Geometry check sheet. Reference: drawing and pictorial views, mm from the part's lowest x, y, z. A direction names the side the tool comes from. Round coordinates to 2 decimals unless told otherwise and drop trailing zeros. Write each loop counter-clockwise with the first axis right and the second up, starting at its lowest first coordinate (ties: lowest second). Pieces come first, ordered by that corner, then holes. Notation, with made-up numbers: (14.25, 5.25) -> (55.25, 5.25) arc R14 ccw to (55.25, 12.25) -> close; hole circle Ø8 at (-1.75, 4.5). An arc over 180 degrees is marked (long way). Write item = value, one per line.
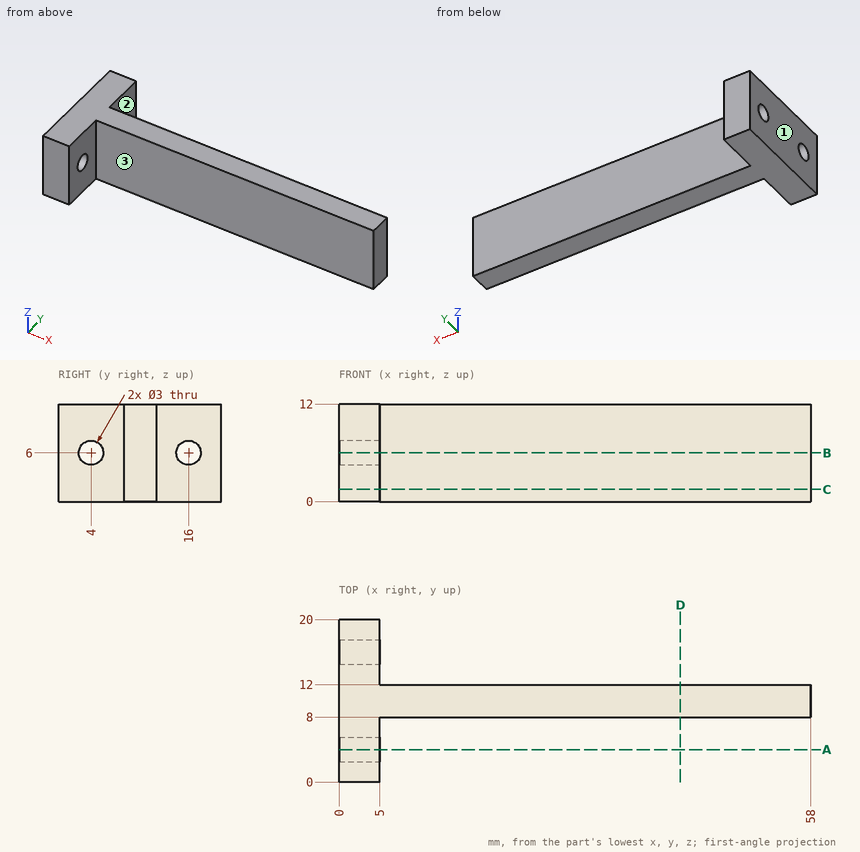
(1) Go/stop test with flat-tipped pins: P1, Ø1.5, axis at x = 44.5, z = 7.5, coming from the -Y side; P2, Ø6.5, axis at y = 2.5, z = 4, coming from the +X side; P3, Ø1, axis at y = 16.5, z = 6, coming from the +X side; P4, Ø6, axis at x = 21.5, z = 5.5, coming from the +Y side. Record where each tip stops, or that it passes through.
Worked answers:
P1 = 8
P2 = 5
P3 = through
P4 = 12
(2) Sectioned sample at D-D on x = 42. Enter the section's corners in (y, z), then the cut area to 3 significant figures.
Worked answers:
outline = (8, 0) -> (12, 0) -> (12, 12) -> (8, 12) -> close
area = 48.0 mm²
(3) Sectioned sample at A-A on y = 4. Enter the section's corners in (x, z).
Worked answers:
outline = (0, 0) -> (5, 0) -> (5, 4.5) -> (0, 4.5) -> close; (0, 7.5) -> (5, 7.5) -> (5, 12) -> (0, 12) -> close
(4) Sectioned sample at C-C on z = 1.5. Enter the section's corners in (x, y), then the cut area to 3 significant figures.
Worked answers:
outline = (0, 0) -> (5, 0) -> (5, 8) -> (58, 8) -> (58, 12) -> (5, 12) -> (5, 20) -> (0, 20) -> close
area = 312 mm²
(5) Sectioned sample at B-B on z = 6. Enter the section's corners in (x, y).
Worked answers:
outline = (0, 0) -> (5, 0) -> (5, 2.5) -> (0, 2.5) -> close; (0, 5.5) -> (5, 5.5) -> (5, 8) -> (58, 8) -> (58, 12) -> (5, 12) -> (5, 14.5) -> (0, 14.5) -> close; (0, 17.5) -> (5, 17.5) -> (5, 20) -> (0, 20) -> close
(6) Access from +Z, -Z, +X, -X, +Y, -Y to the whole of each face (thin tool, end or side, straight path). Record for the marked faces 1, 2 and 3.
Worked answers:
face_1 = +Z, -Z, -X, +Y, -Y
face_2 = +Z, -Z, +X, +Y
face_3 = +Z, -Z, +X, -Y
(7) Material ranges on L1, parallel to Y at x = 2.6, z = 6; L2, parallel to Y at x = 42.5, z = 2; L3, parallel to X at y = 6, z = 9.75, recorded low to high. Write a range as [from, to].
Worked answers:
L1 = [0, 2.5], [5.5, 14.5], [17.5, 20]
L2 = [8, 12]
L3 = [0, 5]
